from build123d import *

# Parameters (mm, degrees)
F0_W     = 27.675628
F0_H     = 25.008082
F1_DEPTH = 46.487905
F2_T     = -4
F3_R     = 6.965851
F4_DEPTH = 39.263487
F5_R     = 6.228625
F6_DEPTH = 30


with BuildPart() as f1:
    # F0 (on Top) → F1 (new body)
    with BuildSketch(Plane.XY):
        Rectangle(F0_W, F0_H)
    extrude(amount=F1_DEPTH)

    # F2
    f2_openings = [f1.faces().sort_by_distance(p)[0] for p in [
        (0, 0, 46.487905),
    ]]
    offset(amount=F2_T, openings=f2_openings)

    # F3 (on Front) → F4 (cut, symmetric)
    with BuildSketch(Plane.XZ):
        with Locations((0, 16.891949)):
            Circle(F3_R)
    extrude(amount=F4_DEPTH, both=True, mode=Mode.SUBTRACT)

    # F5 (on face) → F6 (cut, symmetric)
    with BuildSketch(Plane.YZ.offset(13.837814)):
        with Locations((0, 30.998062)):
            Circle(F5_R)
    extrude(amount=F6_DEPTH, both=True, mode=Mode.SUBTRACT)


solid = f1.part
Can you work these out from the model? Positions are in its coordinate system, mm. A direction names the side the tool comes from. Coordinates: 2 decimals unless noted, no trailing zeros. Order: outer loops, then holes, each group sorted by start corner. A loop starts at its lowest first (then second) coordinate and runs counter-clockwise, first axis right, second up. Notation, with made-up numbers: M 65,10.5 L 110,10.5 A21 ccw 110,16.5 Z; hole C 80.5,13 d1. An arc over 180 degrees is marked long. Answer as CSV lines item,"result".
(1) Suppose I cut it at A-A on y = 0. Please give me the cut outline in (x, z).
Geometry check:
outline,"M -13.84,0 L 13.84,0 L 13.84,24.77 L 9.84,24.77 L 9.84,4 L -9.84,4 L -9.84,24.77 L -13.84,24.77 Z; M -13.84,37.23 L -9.84,37.23 L -9.84,46.49 L -13.84,46.49 Z; M 9.84,37.23 L 13.84,37.23 L 13.84,46.49 L 9.84,46.49 Z"
(2) Please list where these lines run through material, in increasing order: L1, parallel to Y at x = -2.5, z = 41; L2, parallel to Z at x = 0, y = 10.6; L3, parallel to X at y = -4, z = 11.5.
Geometry check:
L1,"-12.5 to -8.5, 8.5 to 12.5"
L2,"0 to 9.93, 23.86 to 46.49"
L3,"-13.84 to -9.84, 9.84 to 13.84"
(3) I'm going to push flat-ended pins straight in: pin 1 (5 mm diameter, centred on x = 6, y = -4, fed in from +Z); pin 2 (10 mm diameter, centred on y = -1, z = 32.5, fed in from +X). Where does each tip first touch, or does it pass through?
Geometry check:
pin 1,"z = 4"
pin 2,"x = 13.84"
(4) Suppose I cut it at D-D on x = -8. Please give me the cut outline in (y, z), plus the area to 3 significant figures.
Geometry check:
outline,"M -12.5,0 L 12.5,0 L 12.5,46.49 L 8.5,46.49 L 8.5,4 L -8.5,4 L -8.5,46.49 L -12.5,46.49 Z"
area,"440 mm^2"
(5) If we mould it in two halves opening along X, with no side actions, what happens to faces 3 (the cylindrical face through (-1.51, 10.48, 10.09)), 4 (the flat face through (-13.838, 0, 23)), 5 (the cylindrical face through (11.866, -0.811, 37.174))? For each: released by +X, released by -X, zero draft, split by the parting line, or undercut.
Geometry check:
face 3,"undercut"
face 4,"released by -X"
face 5,"zero draft"
(6) On a 3-axis mill with a long thin cutter (end or side, diameter ignored), from which of +Z, -Z, +X, -X, +Y, -Y can I reach the whole of each face in a straight line? I mean faces 1 (the flat face through (9.838, -2, 24.9)), 2 (the flat face through (0, 0, 0)). Say none if no direction works.
Geometry check:
face 1,"+Z"
face 2,"-Z, +X, -X, +Y, -Y"
(7) Suppose I cut it at C-C on z = 38. Please give me the cut outline in (x, y).
Geometry check:
outline,"M -13.84,-12.5 L 13.84,-12.5 L 13.84,12.5 L -13.84,12.5 Z; hole M -9.84,-8.5 L 9.84,-8.5 L 9.84,8.5 L -9.84,8.5 Z"
(8) Suppose I cut it at B-B on x = 0. Please give me the cut outline in (y, z).
Geometry check:
outline,"M -12.5,0 L 12.5,0 L 12.5,9.93 L 8.5,9.93 L 8.5,4 L -8.5,4 L -8.5,9.93 L -12.5,9.93 Z; M -12.5,23.86 L -8.5,23.86 L -8.5,46.49 L -12.5,46.49 Z; M 8.5,23.86 L 12.5,23.86 L 12.5,46.49 L 8.5,46.49 Z"
